The model under review builds one solid part; all positions refer to its coordinate system, in mm. A direction names the side the tool comes from. Give positions to 0.01 mm unless a question says otherwise; leave off trailing zeros. Write each loop counter-clockwise with the first axis right and the second up, starting at its lowest first coordinate (ties: lowest second). Pieces come first, ordered by that corner, then holes.
Autodesk Inventor part; units mm, degrees
ref_plane "YZ Plane" through (0, 0, 0) normal (1, 0, 0) x (0, 1, 0)
ref_plane "XZ Plane" through (0, 0, 0) normal (0, 1, 0) x (-1, 0, 0)
ref_plane "XY Plane" through (0, 0, 0) normal (0, 0, 1) x (1, 0, 0)
sketch "Sketch1" plane through (0, 0, 0) normal (0, 1, 0) x (-1, 0, 0)
  circle A0 centre (0, 0) radius 7.5
  dimension "d0" = 15
extrude "Extrusion1" add sketch "Sketch1" along normal blind 2
sketch "Sketch2" plane through (0, 0, 0) normal (0, -1, 0) x (1, 0, 0)
  circle A0 centre (0, 0) radius 4.5
extrude "Extrusion2" add sketch "Sketch2" along normal blind 68
sketch "Sketch4" plane through (0, 2, 0) normal (0, 1, 0) x (1, 0, 0)
  circle A0 centre (0, 0) radius 4.5
  circle A1 centre (0, 0) radius 4.5
  line L0 (-1.6, -4.2059) -> (-1.6, 4.2059)
  line L1 (1.6, -4.2059) -> (1.6, 4.2059)
  dimension "d6" = 9
extrude "Extrusion3" cut sketch "Sketch4" against normal blind 42 contours L1 A0 L0
sketch "Sketch5" plane through (0, 2, 0) normal (0, 1, 0) x (1, 0, 0)
  circle A0 centre (0, 0) radius 4.5
  arc A1 (-1.6, -4.2059) -> (1.6, -4.2059) centre (0, 0) ccw
  line L0 (-1.6, -4.2059) -> (-1.6, 4.2059)
  line L1 (-1.6, -4.2059) -> (-1.6, 4.2059)
  line L2 (1.6, 4.2059) -> (1.6, -4.2059)
  arc A2 (1.6, 4.2059) -> (-1.6, 4.2059) centre (0, 0) ccw
  line L3 (1.6, -4.2059) -> (1.6, 4.2059)
  dimension "d9" = 9
extrude "Extrusion4" add sketch "Sketch5" against normal blind 32 contours L2 A0 L0
fillet "Fillet1" radius 1.5 1 edges at (-1.6, -40, 0)
fillet "Fillet2" radius 1.499 1 edges at (1.6, -40, 0)
sketch "Sketch6" plane through (0, -40, 0) normal (0, 1, 0) x (1, 0, 0)
  point P0 (0, 0)
ref_plane "Work Plane2" through (0.101, -40, -4.4989) normal (0.0224, 0, -0.9997) x (0, 1, 0)
sketch "Sketch8" plane through (0, -68, 0) normal (0, -1, 0) x (1, 0, 0)
  circle A0 centre (0, 0) radius 2.875
  circle A1 centre (0, 0) radius 4.5
  dimension "d23" = 5.75
extrude "Extrusion5" cut sketch "Sketch8" against normal blind 12
sketch "Sketch9" plane through (0.101, -40, -4.4989) normal (0.0224, 0, -0.9997) x (0, 1, 0)
  line L0 (-16, -4.5) -> (-16, 4.5)
  line L1 (-16, 0) -> (10, -0.0944)
  line L2 (10, 1.5052) -> (10, -1.694)
  point P0 (40, 0)
properties part number "pin"
1) Consider section B-B, the plane y = -27.5. Give the boundary of the cut face in (x, z), then the cut area to 3 significant figures.
2) Consider section A-A, the plane z = 0. Give the boundary of the cut face in (x, y) (3 decimals).
3) Tool access review of faces 5 (the flat face through (1, -56, -3)), 6 (the flat face through (1.6, -34, 0)), 7 (the cylindrical face through (7.493, 0.986, -0.33)): name each direction out of +Z, -Z, +X, -X, +Y, -Y from which nothing blocks a thin tool from reaching the whole face with its end or side.
4) To check wall thickness, follow probe 1 along Y at (x, z) = (0.25, -2.5); probe 2 along Y at (x, z) = (-0.5, 6.75); probe 3 along Y at (x, z) = (-3.5, -1.25). State the ranges of each line that lie inside material, in increasing order.
5) Insertion check: pin 1 (8 mm diameter, centred on y = -26, z = 4, fed in from -X); pin 2 (1.5 mm diameter, centred on x = 1, y = -37.5, fed in from +Z); pin 3 (2.5 mm diameter, centred on y = -33, z = 1.5, fed in from +X); pin 4 (1.5 mm diameter, centred on y = -22.5, z = -5.5, fed in from +X). Each pin has a flat end and moves straight along its axis. Give the tip position at first contact, or say it passes through.
6) The part is to be moulded in two halves that separate along X. For faces 1 (the cylindrical face through (4.292, -27.608, -1.352)), 2 (the flat face through (0, 0, -5)), 3 (the flat face through (0, -30, 0)), 4 (the flat face through (-1.6, -34, 0)), say which applies: +X half, -X half, draft (parallel to the pull), parting line (faces both ways), or undercut.
Answer block:
1. outline: circle Ø9 at (0, 0)
1. area: 63.6 mm2
2. outline: (-7.5, 0) - (-4.5, 0) - (-4.5, -56) - (-2.875, -56) - (-2.875, -68) - (2.875, -68) - (2.875, -56) - (4.5, -56) - (4.5, 0) - (7.5, 0) - (7.5, 2) - (-7.5, 2) - close; hole (-1.6, -38.5) arc R1.5 ccw to (-0.1, -40) - (0.101, -40) arc R1.499 ccw to (1.6, -38.501) - (1.6, -30) - (-1.6, -30) - close
3. face 5: -Y
3. face 6: +Z, -Z
3. face 7: +Y, -Y
4. probe 1: y = -68 to -39.99, -30 to 2
4. probe 2: y = 0 to 2
4. probe 3: y = -56 to 2
5. pin 1: stops at x = -4.5
5. pin 2: stops at z = 4.21
5. pin 3: stops at x = 4.49
5. pin 4: passes through
6. face 1: parting line
6. face 2: draft
6. face 3: undercut
6. face 4: undercut
